Can you work these out from the model? Positions are in its coordinate system, mm. A direction names the side the tool comes from. Coordinates: 2 decimals unless noted, no trailing zeros. Order: outer loops, then holes, each group sorted by start corner. A loop starts at its lowest first (then second) coordinate and runs counter-clockwise, first axis right, second up. Notation, with made-up numbers: (-4, -20.75) -> (14, -20.75) arc R21 cw to (14, -1.75) -> close; hole circle Ø8 at (-25.5, 70.5). An arc over 180 degrees is marked (long way). Answer in a Markdown table with one row per item. Add a question column.
1. Imagine slicing it at B-B on y = 5.5. Write out the boundary of the cut face in (x, z), plus the area to 3 significant figures.
2. If I drill on line 1 along Y through (x, z) = (0.75, -2.4); line 2 along X through (y, z) = (15.25, -1.4); line 3 along X through (y, z) = (17.5, -0.45), over which ranges is the centre line in solid material (lowest first)? Write a range as [from, to].
3. Will these pins go through, and if not, where does the flat tip stop? pin 1 (1.5 mm diameter, centred on x = 0.5, z = -1.5, fed in from -Y); pin 2 (1 mm diameter, centred on y = 2.5, z = -2.5, fed in from -X).
4. Imagine slicing it at A-A on x = 0. Write out the boundary of the cut face in (y, z).
5. On a 3-axis mill with a long thin cutter (end or side, diameter ignored), from which of +Z, -Z, +X, -X, +Y, -Y can I reach the whole of each face in a straight line? I mean faces 4 (the face through (0, 12.3, -1.6)), 5 (the face through (4.073, 4.521, -1.914)), 6 (the face through (0, 15, -3)). Say none if no direction works.
6. Imagine slicing it at C-C on y = 8.5. Write out the boundary of the cut face in (x, z).
7. We'd pull the mould along X, two halves only. Please class faces 1 (the face through (0.036, 0.854, -1.639)), 2 (the face through (0, 6, -3)), 3 (the face through (0.017, 2.142, -0.765)): pulls with the +X half, pulls with the -X half, needs draft (parallel to the pull), parting line crosses it, or undercut.
from build123d import *

# Parameters (mm, degrees)
SKETCH001_R     = 0.25
POCKET_DEPTH    = 5
SKETCH002_W     = 10
SKETCH002_H     = 2.096101
SKETCH002_H_2   = 2.304512
POCKET001_DEPTH = 22.001
FILLET_R        = 0.35
SKETCH003_W     = 20
SKETCH003_H     = 10
POCKET002_DEPTH = 22.001


with BuildPart() as part:
    # Sketch → Revolution (revolve)
    with BuildSketch(Plane.XY):
        Polygon((0, 0), (0.5, 0), (4.5, 3), (4.5, 6), (3, 6), (2.454, 6), (2.454, 7), (3, 7), (3, 22), (1.6, 22), (1.6, 2.842559), (0, 1.5), align=None)
    revolve(axis=Axis((0, 0, 0), (0, 1, 0)))

    # Sketch001 → Pocket (cut)
    with BuildSketch(Plane.XZ):
        Circle(SKETCH001_R)
    extrude(amount=-POCKET_DEPTH, mode=Mode.SUBTRACT)

    # Sketch002 → Pocket001 (cut, through all)
    with BuildSketch(Plane.XZ):
        with Locations((-0.418938, 4.548051)):
            Rectangle(SKETCH002_W, SKETCH002_H)
        with Locations((-0.456429, -4.652256)):
            Rectangle(SKETCH002_W, SKETCH002_H_2)
    extrude(amount=-POCKET001_DEPTH, mode=Mode.SUBTRACT)

    # Fillet
    fillet_edges = [part.edges().sort_by_distance(p)[0] for p in [
        (-2.454, 7, 0),
        (-2.454, 6, 0),
    ]]
    fillet(fillet_edges, radius=FILLET_R)

    # Sketch003 → Pocket002 (cut, through all)
    with BuildSketch(Plane(origin=(0, 22, 0), x_dir=(-1, 0, 0), z_dir=(0, 1, 0))):
        with Locations((0, 5)):
            Rectangle(SKETCH003_W, SKETCH003_H)
    extrude(amount=-POCKET002_DEPTH, mode=Mode.SUBTRACT)


solid = part.part
Answers follow:
| question | item | result |
|---|---|---|
| 1 | outline | (-4.5, 0) arc R4.5 ccw to (-2.83, -3.5) -> (2.83, -3.5) arc R4.5 ccw to (4.5, 0) -> (1.6, 0) arc R1.6 cw to (-1.6, 0) -> close |
| 1 | area | 23.9 mm² |
| 2 | line 1 | y = [1.51, 6.15], [6.85, 22] |
| 2 | line 2 | x = [-2.65, -0.77], [0.77, 2.65] |
| 2 | line 3 | x = [-2.97, -1.54], [1.54, 2.97] |
| 3 | pin 1 | stops at y = 0.25 |
| 3 | pin 2 | stops at x = -3.8 |
| 4 | outline | (0, -0.5) -> (2.25, -3.5) -> (6, -3.5) -> (6, -2.8) arc R0.35 cw to (6.35, -2.45) -> (6.65, -2.45) arc R0.35 cw to (7, -2.8) -> (7, -3) -> (22, -3) -> (22, -1.6) -> (2.84, -1.6) -> (1.71, -0.25) -> (0, -0.25) -> close |
| 5 | face 4 | +Z, +Y |
| 5 | face 5 | -Z, +X, +Y, -Y |
| 5 | face 6 | -Z, +Y |
| 6 | outline | (-3, 0) arc R3 ccw to (3, 0) -> (1.6, 0) arc R1.6 cw to (-1.6, 0) -> close |
| 7 | face 1 | parting line crosses it |
| 7 | face 2 | needs draft |
| 7 | face 3 | undercut |
